Part model, mm, in its own coordinate system. A direction names the side the tool comes from. Round coordinates to 2 decimals unless told otherwise and drop trailing zeros. Write each loop counter-clockwise with the first axis right and the second up, starting at its lowest first coordinate (ties: lowest second). Pieces come first, ordered by that corner, then holes.
1) Saw through at C-C on y = -11. Write the cut outline in (x, z).
2) Saw through at D-D on z = 56.5. Write the cut outline in (x, y).
3) Flat gauge pin, fed straight in: pin 1 (2.5 mm diameter, centred on x = 31.5, y = 7, fed in from +Z). Where does the tip first touch, or does it go through?
4) Which spindle directions (+Z, -Z, +X, -X, +Y, -Y) get a long thin tool onto all of the face, cutting with end or side? Do faces 1 (the flat face through (-27.532, -1, 444)), 2 (the flat face through (-30.532, -2, 444)). Say none if no direction does.
5) Pull direction Z, two halves, no side cores. Call faces 3 (the flat face through (-30, -1, 900)), 4 (the cylindrical face through (-0.949, -31.348, 46.738)), 5 (the flat face through (-1, -32, 0)), 6 (the flat face through (1, 30.673, 444)): +Z half, -Z half, draft (parallel to the pull), parting line (faces both ways), or undercut.
6) Saw through at B-B on z = 733.5. Write the cut outline in (x, y), and give its area (3 significant figures).
7) Saw through at A-A on x = 21. Write the cut outline in (y, z).
8) Drill centre lines: L1, parallel to Y at x = -25, z = 670.5; L2, parallel to X at y = 15, z = 55. Where is each one in solid material? Low to high.
```python
from build123d import *

# Parameters (mm, degrees)
F0_W     = 63.5
F0_H     = 63.5
F0_W_2   = 57.5
F0_H_2   = 57.5
F1_DEPTH = 900
F2_W     = 57.5
F2_H     = 53.5
F3_DEPTH = 3
F4_R     = 10
F5_DEPTH = 3


with BuildPart() as f1:
    # F0 (on Top) → F1 (new body)
    with BuildSketch(Plane.XY):
        with Locations((1.218427, -1.076905)):
            Rectangle(F0_W, F0_H)
        with Locations((1.218427, -1.076905)):
            Rectangle(F0_W_2, F0_H_2, mode=Mode.SUBTRACT)
    extrude(amount=F1_DEPTH)

    # F2 (on face) → F3 (cut)
    with BuildSketch(Plane.YZ.offset(32.968427)):
        with Locations((-1.076905, 873.25)):
            Rectangle(F2_W, F2_H)
    extrude(amount=-F3_DEPTH, mode=Mode.SUBTRACT)

    # F4 (on face) → F5 (cut)
    with BuildSketch(Plane.XZ.offset(32.826905)):
        with Locations((1.218427, 56.5)):
            Circle(F4_R)
    extrude(amount=-F5_DEPTH, mode=Mode.SUBTRACT)


solid = f1.part
```
Completed:
1. outline: (-30.53, 0) - (-27.53, 0) - (-27.53, 900) - (-30.53, 900) - close; (29.97, 0) - (32.97, 0) - (32.97, 846.5) - (29.97, 846.5) - close
2. outline: (-30.53, -32.83) - (-8.78, -32.83) - (-8.78, -29.83) - (-27.53, -29.83) - (-27.53, 27.67) - (29.97, 27.67) - (29.97, -29.83) - (11.22, -29.83) - (11.22, -32.83) - (32.97, -32.83) - (32.97, 30.67) - (-30.53, 30.67) - close
3. pin 1: stops at z = 846.5
4. face 1: +Z, -Z
4. face 2: +Z, -Z, -X, +Y, -Y
5. face 3: +Z half
5. face 4: undercut
5. face 5: -Z half
5. face 6: draft
6. outline: (-30.53, -32.83) - (32.97, -32.83) - (32.97, 30.67) - (-30.53, 30.67) - close; hole (-27.53, -29.83) - (29.97, -29.83) - (29.97, 27.67) - (-27.53, 27.67) - close
6. area: 726 mm2
7. outline: (-32.83, 0) - (-29.83, 0) - (-29.83, 900) - (-32.83, 900) - close; (27.67, 0) - (30.67, 0) - (30.67, 900) - (27.67, 900) - close
8. L1: y = -32.83 to -29.83, 27.67 to 30.67
8. L2: x = -30.53 to -27.53, 29.97 to 32.97
